from build123d import *

# Parameters (mm, degrees)
EXTRUDE_1_DEPTH    = 755
SKETCH_4_W         = 8
SKETCH_4_H         = 20
SKETCH_4_R         = 1.5
EXTRUDE_2_DEPTH    = 2
FILLET_1_R         = 8
SKETCH_5_W         = 4
SKETCH_5_H         = 1.5
EXTRUDE_3_DEPTH    = 5
HOLE_WIZARD_M3_2_D = 2.5


with BuildPart() as part:
    # 草图1 → 凸台-拉伸1 (new body)
    with BuildSketch(Plane.XY):
        Polygon((0.29532044, 2.240431683), (8.29532044, 2.240431683), (8.29532044, 8.240431683), (6.29532044, 8.240431683), (6.29532044, 4.740431683), (2.29532044, 4.740431683), (2.29532044, 14.740431683), (6.29532044, 14.740431683), (6.29532044, 12.240431683), (8.29532044, 12.240431683), (8.29532044, 14.740431683), (8.29532044, 17.240431683), (0.29532044, 17.240431683), align=None)
    extrude(amount=EXTRUDE_1_DEPTH)

    # 草图4 → 凸台-拉伸2 (add)
    # profile 1 of 3: a face of its own
    with BuildSketch(Plane(origin=(0, 2.240431683, 0), x_dir=(-1, 0, 0), z_dir=(0, -1, 0))):
        with Locations((-12.29532044, -689.500000045)):
            Rectangle(SKETCH_4_W, SKETCH_4_H)
        with Locations(Location((-12.29532044, -689.500000045, 0), (0, 0, 90))):
            Circle(SKETCH_4_R, mode=Mode.SUBTRACT)
    # profile 2 of 3: a face of its own
    with BuildSketch(Plane(origin=(0, 2.240431683, 0), x_dir=(-1, 0, 0), z_dir=(0, -1, 0))):
        with Locations((-12.29532044, -399.500000045)):
            Rectangle(SKETCH_4_W, SKETCH_4_H)
        with Locations(Location((-12.29532044, -399.500000045, 0), (0, 0, 90))):
            Circle(SKETCH_4_R, mode=Mode.SUBTRACT)
    # profile 3 of 3: a face of its own
    with BuildSketch(Plane(origin=(0, 2.240431683, 0), x_dir=(-1, 0, 0), z_dir=(0, -1, 0))):
        with Locations((-12.29532044, -69.500000045)):
            Rectangle(SKETCH_4_W, SKETCH_4_H)
        with Locations(Location((-12.29532044, -69.500000045, 0), (0, 0, 90))):
            Circle(SKETCH_4_R, mode=Mode.SUBTRACT)
    extrude(amount=-EXTRUDE_2_DEPTH)

    # 圆角1
    fillet_1_edges = [part.edges().sort_by_distance(p)[0] for p in [
        (8.29532044, 3.240431683, 79.500000045),
        (8.29532044, 3.240431683, 59.500000045),
        (8.29532044, 3.240431683, 389.500000045),
        (8.29532044, 3.240431683, 409.500000045),
        (8.29532044, 3.240431683, 679.500000045),
        (8.29532044, 3.240431683, 699.500000045),
    ]]
    fillet(fillet_1_edges, radius=FILLET_1_R - 0.0001)  # a hair under: the kernel refuses the full size

    # 草图5 → 凸台-拉伸3 (add)
    with BuildSketch(Plane.XY.offset(755)):
        with Locations((4.29532044, 5.490431683)):
            Rectangle(SKETCH_5_W, SKETCH_5_H)
    extrude_3 = extrude(amount=-EXTRUDE_3_DEPTH)

    # M3 螺纹孔2 (through all)
    with Locations(Plane(origin=(8.29532044, 0, 0), x_dir=(0, 0, -1), z_dir=(1, 0, 0))):
        with Locations((-752, 4.740431683)):
            hole_wizard_m3_2 = Hole(HOLE_WIZARD_M3_2_D / 2)

    # 镜向1: 凸台-拉伸3, M3 螺纹孔2 across plane
    add(extrude_3.mirror(Plane(origin=(0, 0, 377.5), x_dir=(1, 0, 0), z_dir=(0, 0, -1))))
    add(hole_wizard_m3_2.mirror(Plane(origin=(0, 0, 377.5), x_dir=(1, 0, 0), z_dir=(0, 0, -1))), mode=Mode.SUBTRACT)


solid = part.part
CAD build for the part. Positions are in the model's coordinates, mm. Round coordinates to 2 decimals unless told otherwise and drop trailing zeros. Order: outer loops, then holes, each group sorted by start corner. A loop starts at its lowest first (then second) coordinate and runs counter-clockwise, first axis right, second up. Notation, with made-up numbers: M 24,32.5 L 67,32.5 A18 cw 67,62.5 Z; hole C 25.5,75 d9. An arc over 180 degrees is marked long. Use one line per item in the form item = value.
Q1. Flat gauge pins, fed straight in: P1, Ø1.5, axis at y = 4.74, z = 752, coming from the -X side; P2, Ø1.8, axis at y = 4.5, z = 433.5, coming from the +X side; P3, Ø3.5, axis at x = 12.3, z = 399.5, coming from the +Y side; P4, Ø3, axis at y = 10.5, z = 396, coming from the +X side. Where does each tip first touch, or does it go through?
Recorded:
P1 = through
P2 = 8.3
P3 = 4.24
P4 = 2.3
Q2. Saw through at A-A on z = 440. Give the cut face in (x, y).
Recorded:
outline = M 0.3,2.24 L 8.3,2.24 L 8.3,8.24 L 6.3,8.24 L 6.3,4.74 L 2.3,4.74 L 2.3,14.74 L 6.3,14.74 L 6.3,12.24 L 8.3,12.24 L 8.3,17.24 L 0.3,17.24 Z
Q3. Probe L1, parallel to Y at x = 2.75, z = 752; L2, parallel to X at y = 3.65, z = 69.5; L3, parallel to Z at x = 1.75, y = 4.5. List the from-to ranges inside material, lowest first.
Recorded:
L1 = 2.24 to 3.49, 5.99 to 6.24, 14.74 to 17.24
L2 = 0.3 to 10.8, 13.8 to 16.3
L3 = 0 to 1.77, 4.23 to 750.77, 753.23 to 755
